Verification items for the finished model (mm, model axes). Face numbers are marked on the shaded views. A direction names the side the tool comes from. Round coordinates to 2 decimals unless told otherwise and drop trailing zeros. Order: outer loops, then holes, each group sorted by start corner. A loop starts at its lowest first (then second) coordinate and runs counter-clockwise, first axis right, second up. Notation, with made-up numbers: M -10,-14.75 L 5,-14.75 A23 ccw 5,23.25 Z; hole C 42,32.25 d1. An arc over 180 degrees is marked long. Write item = value, one per line. Start each with the question number.
from build123d import *

# Parameters (mm, degrees)
F0_R          = 7.5
F1_DEPTH      = 115
F2_SIZE2      = 1
F2_SIZE       = 1
F3_W          = 1.5
F3_H          = 10
F4_DEPTH      = 7.501
F4_DEPTH_BACK = 7.501


with BuildPart() as f1:
    # F0 (on Top) → F1 (new body)
    with BuildSketch(Plane.XY):
        Circle(F0_R)
    extrude(amount=F1_DEPTH)

    # F2
    f2_edges = [f1.edges().sort_by_distance(p)[0] for p in [
        (-7.5, 0, 115),
        (-7.5, 0, 0),
    ]]
    chamfer(f2_edges, length=F2_SIZE, length2=F2_SIZE2)

    # F3 (on Front) → F4 (cut, two sides)
    with BuildSketch(Plane.XZ) as f4_sk:
        with Locations((6.75, 13)):
            Rectangle(F3_W, F3_H)
        with Locations((-6.75, 13)):
            Rectangle(F3_W, F3_H)
    extrude(amount=F4_DEPTH, mode=Mode.SUBTRACT)
    extrude(f4_sk.sketch, amount=-F4_DEPTH_BACK, mode=Mode.SUBTRACT)


solid = f1.part
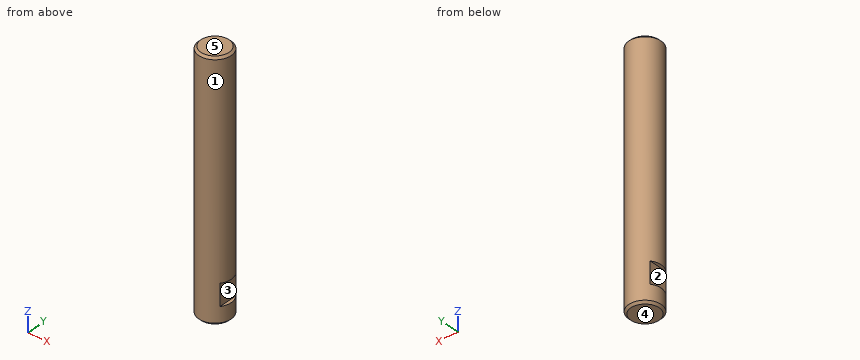
1) Gauge pin test, flat ends, axial feed: P1, Ø3, axis at y = 1, z = 79.5, coming from the -X side; P2, Ø4.5, axis at y = -0.5, z = 15, coming from the -X side; P3, Ø2, axis at x = -5.5, z = 51.5, coming from the +Y side; P4, Ø1.5, axis at y = -4, z = 30.5, coming from the +X side. Record the tip position at first contact, or that the pin passes through.
2) Cross-section at A-A, the plane y = 0. Enter the section's corners in (x, z), then the cut area to 3 significant figures.
3) Access from +Z, -Z, +X, -X, +Y, -Y to the whole of each face (thin tool, end or side, straight path). Record for the marked faces 1 and 2.
4) Scan lines: probe 1 along Y at (x, z) = (-0.5, 27); probe 2 along Y at (x, z) = (4.5, 98); probe 3 along Z at (x, y) = (-2, 6.25). Record each from-to range of solid material in increasing order.
5) Release check for a two-part mould opening along Z. For the marked faces 3, 4 and 5 record: pulls with the +Z half, pulls with the -Z half, needs draft (parallel to the pull), parting line crosses it, or undercut.
6) Cross-section at B-B, the plane z = 23.5. Enter the section's corners in (x, y), then the cut area to 3 significant figures.
Geometry results:
q1.P1 = -7.5
q1.P2 = -6
q1.P3 = 6
q1.P4 = 6.76
q2.outline = M -7.5,1 L -6.5,0 L 6.5,0 L 7.5,1 L 7.5,8 L 6,8 L 6,18 L 7.5,18 L 7.5,114 L 6.5,115 L -6.5,115 L -7.5,114 L -7.5,18 L -6,18 L -6,8 L -7.5,8 Z
q2.area = 1,690 mm^2
q3.face_1 = +Z, -Z
q3.face_2 = -X, +Y, -Y
q4.probe_1 = -7.48 to 7.48
q4.probe_2 = -6 to 6
q4.probe_3 = 0.06 to 114.94
q5.face_3 = undercut
q5.face_4 = pulls with the -Z half
q5.face_5 = pulls with the +Z half
q6.outline = C 0,0 d15
q6.area = 177 mm^2
